Autodesk Inventor part; units mm, degrees
ref_plane "YZ Plane" through (0, 0, 0) normal (1, 0, 0) x (0, 1, 0)
ref_plane "XZ Plane" through (0, 0, 0) normal (0, 1, 0) x (-1, 0, 0)
ref_plane "XY Plane" through (0, 0, 0) normal (0, 0, 1) x (1, 0, 0)
sketch "Sketch1" plane through (0, 0, 0) normal (0, 0, 1) x (1, 0, 0)
  circle A0 centre (0, 0) radius 6.2
  line L0 (0, 0) -> (83.2978, 0) construction
  circle A1 centre (37, 0) radius 2.6
  line L1 (-10, 10) -> (47, 10)
  line L2 (47, 10) -> (47, -15)
  line L3 (47, -15) -> (-10, -15)
  line L4 (-10, -15) -> (-10, 10)
  line L5 (22, 29.5766) -> (22, -18.8569) construction
  dimension "d0" = 12.4
  dimension "d1" = 5.2
  dimension "d2" = 37
  dimension "d3" = 10
  dimension "d4" = 15
  dimension "d5" = 10
  dimension "d6" = 22
  dimension "d7" = 25
extrude "Extrusion1" add sketch "Sketch1" along normal blind 5
sketch "Sketch2" plane through (0, 0, 5) normal (0, 0, 1) x (1, 0, 0)
  circle A0 centre (0, 0) radius 6.2
  circle A1 centre (37, 0) radius 2.6
  line L0 (47, 10) -> (-10, 10)
  line L1 (-10, 10) -> (-10, -15)
  line L2 (-10, -15) -> (47, -15)
  line L3 (47, -15) -> (47, 10)
  line L4 (22, 10) -> (22, -15)
  dimension "d10" = 22
extrude "Extrusion2" add sketch "Sketch2" along normal blind 7 contours L4 L2 L1 L0
sketch "Sketch3" plane through (0, 0, 12) normal (0, 0, 1) x (1, 0, 0)
  point P0 (0, 0)
sketch "Sketch4" plane through (0, 0, 5) normal (0, 0, 1) x (1, 0, 0)
  circle A0 centre (0, 0) radius 6.2
  line L0 (-10, 10) -> (-10, -15)
  line L1 (-10, -15) -> (22, -15)
  line L2 (22, -15) -> (22, 10)
  line L3 (22, 10) -> (-10, 10)
  line L4 (22, 10) -> (17, 10)
  line L5 (17, 10) -> (17, -15)
  line L6 (17, -15) -> (22, -15)
  line L7 (22, -15) -> (22, 10)
  dimension "d13" = 5
extrude "Extrusion3" add sketch "Sketch4" along normal blind 25 contours L3 L2 L1 L5
chamfer "Chamfer1" distance 6 angle 45 1 edges at (-10, 10, 6)
chamfer "Chamfer2" distance 2 angle 45 1 edges at (17, -2.5, 12)
chamfer "Chamfer3" distance 11 angle 45 1 edges at (-10, -15, 6)
sketch "Sketch5" plane through (22, -15, 5) normal (1, 0, 0) x (0, 0, -1)
  line L0 (0, 25) -> (0, 0) construction
  line L1 (-9, 0) -> (-25, 0)
  point P0 (5, 15)
  point P1 (-15, 7.5)
  dimension "d22" = 15
  dimension "d62" = 7.5
hole "Hole1" at (22, -7.5, 20) direction (-1, 0, 0) diameter 5.2 end through all
sketch "Sketch6" plane through (0, 0, 5) normal (0, 0, 1) x (1, 0, 0)
  line L0 (22, 10) -> (22, -15)
  line L1 (22, -15) -> (47, -15)
  line L2 (47, -15) -> (47, 10)
  line L3 (47, 10) -> (22, 10)
  circle A0 centre (37, 0) radius 2.6
  line L4 (39.6, 0) -> (39.6, 10)
  circle A1 centre (37, 0) radius 2.6
  line L5 (34.4, 0) -> (34.4, 10)
  line L6 (-4, 10) -> (47, 10)
  circle A2 centre (37, 0) radius 2.6
  point P0 (0, 0)
extrude "Extrusion4" cut sketch "Sketch6" against normal through all contours L3 L4 A0 L5
sketch "Sketch7" plane through (0, 0, 12) normal (0, 0, 1) x (1, 0, 0)
  line L0 (15, 10) -> (15, -15)
  line L1 (15, 10) -> (-4, 10)
  line L2 (-10, 4) -> (-4, 10)
  line L3 (-10, 4) -> (-10, -4)
  line L4 (1, -15) -> (15, -15)
  circle A0 centre (0, 0) radius 6.2
  line L5 (14.25, 10) -> (14.25, 4.25)
  line L6 (14.25, 4.25) -> (4.5141, 4.25)
  line L7 (5.1176, 3.5) -> (15, 3.5)
  line L8 (1, -15) -> (-10, -4)
  dimension "d33" = 0.75
  dimension "d34" = 0.75
  dimension "d35" = 3.5
extrude "Extrusion5" cut sketch "Sketch7" against normal through all contours L0 L7 A0 L6 L5 L1
fillet "Fillet1" radius 0.5 1 edges at (5.1176, 3.5, 6)
fillet "Fillet2" radius 0.5 1 edges at (4.5141, 4.25, 6)
sketch "Sketch8" plane through (-4, 10, 12) normal (0, 1, 0) x (1, 0, 0)
  line L0 (18.25, 0) -> (18.25, 12)
  line L1 (0, 12) -> (18.25, 12)
  line L2 (0, 0) -> (0, 12)
  line L3 (18.25, 0) -> (0, 0)
  point P0 (4, 12)
  point P1 (14, 6)
  dimension "d40" = 10
  dimension "d41" = 6
hole "Hole2" at (10, 10, 6) direction (0, -1, 0) diameter 3.5 end through all
sketch "Sketch9" plane through (47, -15, 0) normal (0, -1, 0) x (1, 0, 0)
  circle A0 centre (-37, 6) radius 1.75
  circle A1 centre (-37, 6) radius 1.75
  point P0 (-47, 0)
  point P1 (-37, 6)
hole "Hole3" at (10, -15, 6) direction (0, 1, 0) diameter 4.7 depth 5 counterbore diameter 5 counterbore depth 0.5
fillet "Fillet4" radius 0.5 8 edges at (34.4, 10, 2.5) (39.6, 10, 2.5) (47, 10, 2.5) (47, -15, 2.5) (22, 10, 17.5) (17, 10, 22) (22, -15, 17.5) (17, -15, 22)
fillet "Fillet5" radius 4 4 edges at (-4, 10, 6) (-10, 4, 6) (-10, -4, 6) (1, -15, 6)
properties part number "Z Axis Linear Rail Bracket - Left 1.0" material "PC/ABS Plastic"
Could you check a few things on this model? Use its own coordinates, in mm. A direction names the side the tool comes from. Round coordinates to 2 decimals unless told otherwise and drop trailing zeros. Write each loop counter-clockwise with the first axis right and the second up, starting at its lowest first coordinate (ties: lowest second). Pieces come first, ordered by that corner, then holes. Notation, with made-up numbers: (60.25, 10.25) - (89.25, 10.25) arc R31 cw to (89.25, 38.25) - close; hole circle Ø3 at (25.25, -6). An arc over 180 degrees is marked (long way). Put each result on its own line as item: value. Start each with the question number.
(1) I want a section at C-C, the plane x = 10. Please give me the cut outline in (y, z), plus the area to 3 significant figures.
(2) Will these pins go through, and if not, where does the flat tip stop? pin 1 (2 mm diameter, centred on y = -5.5, z = 8.5, fed in from +X); pin 2 (4 mm diameter, centred on y = -1, z = 22.5, fed in from -X); pin 3 (12.5 mm diameter, centred on x = 1, y = -4, fed in from +Z).
(3) I need wall thicknesses on probe 1 along Z at (x, y) = (10, -14.75); probe 2 along X at (y, z) = (8.75, 6); probe 3 along Z at (x, y) = (10, -11.1). Which ranges of each line are inside material? Lowest first, please.
(4) I want a section at B-B, the plane y = -7.5. Please give me the cut outline in (x, z), plus the area to 3 significant figures.
(5) I want a section at D-D, the plane z = 20. Please give me the cut outline in (x, y), plus the area to 3 significant figures.
(6) Thinking about a two-plate mould opening in X: for faces 4 (the flat face through (17, -2, 22)), 5 (the flat face through (47, -2, 2)), 6 (the flat face through (21, -15, 7)), 7 (the cylindrical face through (8.265, -3.344, 5.772)), which applies, released by +X, released by -X, zero draft, split by the parting line, or undercut?
(7) I want a section at A-A, the plane y = 7. Please give me the cut outline in (x, z).
(8) For faces 1 (the cylindrical face through (12.22, -14.75, 4.85)), 2 (the flat face through (11.4, 3.5, 7.4)), 3 (the flat face through (34.4, 5, 3)), which set-ups out of +Z, -Z, +X, -X, +Y, -Y let a thin tool reach every point of the face, with its end or its side?
Here are the results:
1. outline: (-15, 0) - (3.5, 0) - (3.5, 4.25) - (-10, 4.25) - (-10, 3.65) - (-14.5, 3.65) - (-14.5, 3.5) - (-15, 3.5) - close; (-15, 8.5) - (-14.5, 8.5) - (-14.5, 8.35) - (-10, 8.35) - (-10, 7.75) - (3.5, 7.75) - (3.5, 12) - (-15, 12) - close; (4.25, 0) - (10, 0) - (10, 4.25) - (4.25, 4.25) - close; (4.25, 7.75) - (10, 7.75) - (10, 12) - (4.25, 12) - close
1. area: 200 mm^2
2. pin 1: stops at x = 22
2. pin 2: stops at x = 17
2. pin 3: stops at z = 12
3. probe 1: z = 0 to 3.5, 8.5 to 12
3. probe 2: x = -5.25 to 8.25, 11.75 to 14.25, 15 to 22
3. probe 3: z = 0 to 3.65, 8.35 to 12
4. outline: (-6.5, 0) - (47, 0) - (47, 5) - (22, 5) - (22, 17.4) - (17, 17.4) - (17, 14) - (15, 12) - (-6.5, 12) - close; (17, 22.6) - (22, 22.6) - (22, 30) - (17, 30) - close; hole circle Ø3.5 at (10, 6)
4. area: 523 mm^2
5. outline: (17, -14.5) arc R0.5 ccw to (17.5, -15) - (21.5, -15) arc R0.5 ccw to (22, -14.5) - (22, -10.1) - (17, -10.1) - close; (17, -4.9) - (22, -4.9) - (22, 9.5) arc R0.5 ccw to (21.5, 10) - (17.5, 10) arc R0.5 ccw to (17, 9.5) - close
5. area: 98.8 mm^2
6. face 4: released by -X
6. face 5: released by +X
6. face 6: zero draft
6. face 7: undercut
7. outline: (-7, 0) - (14.25, 0) - (14.25, 12) - (-7, 12) - close; (15, 0) - (34.4, 0) - (34.4, 5) - (22, 5) - (22, 30) - (17, 30) - (17, 14) - (15, 12) - close; (39.6, 0) - (47, 0) - (47, 5) - (39.6, 5) - close; hole circle Ø3.5 at (10, 6)
8. face 1: -Y
8. face 2: +Z, -Z
8. face 3: +Z, -Z, +Y
